from build123d import *

# Parameters (mm, degrees)
F0_W         = 10.668002069
F0_H         = 8.5344007239
F1_DEPTH     = 25.4
F2_W         = 22.2503971308
F2_H         = 8.5344007239
F2_W_2       = 10.668002069
F3_DEPTH     = 10.16
F4_T1_DEPTH  = 80.5687963307
F4_T3_DEPTH  = 34.9503971308
F4_T5_DEPTH  = 34.9503971308
F4_T10_DEPTH = 47.6503971308
F4_T15_DEPTH = 47.6503971308
F4_T20_DEPTH = 47.6503971308
F4_T25_DEPTH = 47.6503971308


# Not quite as in the source:
# - a fillet or chamfer that OpenCascade refuses, or shapes differently, is made with other operations: its cross-section is extruded or revolved along the edge and cut away or added


with BuildPart() as f1:
    # F0 (on Front) → F1 (new body)
    with BuildSketch(Plane.XZ):
        Rectangle(F0_W, F0_H)
    extrude(amount=F1_DEPTH)

    # F2 (on face) → F3 (join)
    with BuildSketch(Plane(origin=(0, 0, 0), x_dir=(-1, 0, 0), z_dir=(0, 1, 0))):
        with Locations((-16.4591995999, 0)):
            Rectangle(F2_W, F2_H)
        Rectangle(F2_W_2, F2_H)
        with Locations((16.4591995999, 0)):
            Rectangle(F2_W, F2_H)
    extrude(amount=F3_DEPTH)

    # F4: fillet of radius 5.08 on 6 edges, made by hand

    # F4_s2 → F4_t1 (cut)
    with BuildSketch(Plane.YZ.offset(-40.2843981653)):
        with BuildLine():
            ThreePointArc((10.16, -0.8127996381), (8.6721024484, 2.7793028104), (5.08, 4.2672003619))
            Line((5.08, 4.2672003619), (10.16, 4.2672003619))
            Line((10.16, 4.2672003619), (10.16, -0.8127996381))
        make_face()
        with BuildLine():
            ThreePointArc((5.08, -4.2672003619), (8.6721024484, -2.7793028104), (10.16, 0.8127996381))
            Line((10.16, 0.8127996381), (10.16, -4.2672003619))
            Line((10.16, -4.2672003619), (5.08, -4.2672003619))
        make_face()
    extrude(amount=F4_T1_DEPTH, mode=Mode.SUBTRACT)

    # F4_s4 → F4_t3 (cut)
    with BuildSketch(Plane.YZ.offset(5.3340010345)):
        with BuildLine():
            ThreePointArc((0, -0.8127996381), (1.4878975516, 2.7793028104), (5.08, 4.2672003619))
            Line((5.08, 4.2672003619), (0, 4.2672003619))
            Line((0, 4.2672003619), (0, -0.8127996381))
        make_face()
        with BuildLine():
            ThreePointArc((5.08, -4.2672003619), (1.4878975516, -2.7793028104), (0, 0.8127996381))
            Line((0, 0.8127996381), (0, -4.2672003619))
            Line((0, -4.2672003619), (5.08, -4.2672003619))
        make_face()
    extrude(amount=F4_T3_DEPTH, mode=Mode.SUBTRACT)

    # F4_s6 → F4_t5 (cut)
    with BuildSketch(Plane.YZ.offset(-40.2843981653)):
        with BuildLine():
            ThreePointArc((5.08, -4.2672003619), (1.4878975516, -2.7793028104), (0, 0.8127996381))
            Line((0, 0.8127996381), (0, -4.2672003619))
            Line((0, -4.2672003619), (5.08, -4.2672003619))
        make_face()
        with BuildLine():
            ThreePointArc((0, -0.8127996381), (1.4878975516, 2.7793028104), (5.08, 4.2672003619))
            Line((5.08, 4.2672003619), (0, 4.2672003619))
            Line((0, 4.2672003619), (0, -0.8127996381))
        make_face()
    extrude(amount=F4_T5_DEPTH, mode=Mode.SUBTRACT)


with BuildPart() as f4_tool8:
    # F4_s9 → F4_t10 (new body)
    with BuildSketch(Plane.YZ.offset(-7.3659989655)):
        with BuildLine():
            ThreePointArc((0, -0.8127996381), (1.4878975516, 2.7793028104), (5.08, 4.2672003619))
            Line((5.08, 4.2672003619), (0, 4.2672003619))
            Line((0, 4.2672003619), (0, -0.8127996381))
        make_face()
    extrude(amount=F4_T10_DEPTH)

    split(bisect_by=Plane.YZ.offset(-5.3340010345), keep=Keep.BOTTOM)


with BuildPart() as f1_1:
    add(f1.part)

    # F4_t7: cut F4_tool8
    add(f4_tool8.part, mode=Mode.SUBTRACT)


with BuildPart() as f4_tool13:
    # F4_s14 → F4_t15 (new body)
    with BuildSketch(Plane.YZ.offset(40.2843981653)):
        with BuildLine():
            ThreePointArc((5.08, -4.2672003619), (1.4878975516, -2.7793028104), (0, 0.8127996381))
            Line((0, 0.8127996381), (0, -4.2672003619))
            Line((0, -4.2672003619), (5.08, -4.2672003619))
        make_face()
    extrude(amount=-F4_T15_DEPTH)

    split(bisect_by=Plane.YZ.offset(-5.3340010345), keep=Keep.BOTTOM)


with BuildPart() as f1_2:
    add(f1_1.part)

    # F4_t12: cut F4_tool13
    add(f4_tool13.part, mode=Mode.SUBTRACT)


with BuildPart() as f4_tool18:
    # F4_s19 → F4_t20 (new body)
    with BuildSketch(Plane.YZ.offset(7.3659989655)):
        with BuildLine():
            ThreePointArc((5.08, -4.2672003619), (1.4878975516, -2.7793028104), (0, 0.8127996381))
            Line((0, 0.8127996381), (0, -4.2672003619))
            Line((0, -4.2672003619), (5.08, -4.2672003619))
        make_face()
    extrude(amount=-F4_T20_DEPTH)

    split(bisect_by=Plane.YZ.offset(5.3340010345), keep=Keep.TOP)


with BuildPart() as f1_3:
    add(f1_2.part)

    # F4_t17: cut F4_tool18
    add(f4_tool18.part, mode=Mode.SUBTRACT)


with BuildPart() as f4_tool23:
    # F4_s24 → F4_t25 (new body)
    with BuildSketch(Plane.YZ.offset(-40.2843981653)):
        with BuildLine():
            ThreePointArc((0, -0.8127996381), (1.4878975516, 2.7793028104), (5.08, 4.2672003619))
            Line((5.08, 4.2672003619), (0, 4.2672003619))
            Line((0, 4.2672003619), (0, -0.8127996381))
        make_face()
    extrude(amount=F4_T25_DEPTH)

    split(bisect_by=Plane.YZ.offset(5.3340010345), keep=Keep.TOP)


with BuildPart() as f1_4:
    add(f1_3.part)

    # F4_t22: cut F4_tool23
    add(f4_tool23.part, mode=Mode.SUBTRACT)


solid = f1_4.part
Part model, mm, in its own coordinate system. Give positions to 0.01 mm unless a question says otherwise; leave off trailing zeros. Order: outer loops, then holes, each group sorted by start corner. A loop starts at its lowest first (then second) coordinate and runs counter-clockwise, first axis right, second up. Notation, with made-up numbers: (46, 56.5) - (104, 56.5) arc R11 cw to (104, 69.5) - close; hole circle Ø8 at (-33, -3). An arc over 180 degrees is marked (long way). Use a Markdown table: item, result.
1) Saw through at C-C on y = -7. List the corners of the cut face in (x, z), plus the area to 3 significant figures.
Checked values:
| item | result |
|---|---|
| outline | (-5.33, -4.27) - (5.33, -4.27) - (5.33, 4.27) - (-5.33, 4.27) - close |
| area | 91.0 mm² |
2) Saw through at A-A on z = 3. List the corners of the cut face in (x, y).
Checked values:
| item | result |
|---|---|
| outline | (-27.58, 1.72) - (-5.33, 1.72) - (-5.33, -25.4) - (5.33, -25.4) - (5.33, 1.72) - (27.58, 1.72) - (27.58, 8.44) - (-27.58, 8.44) - close |
3) Probe L1, parallel to X at y = -9, z = -3.25; L2, parallel to Y at x = -10.5, z = -1; L3, parallel to Y at x = -20.5, z = 0.5. List the from-to ranges inside material, lowest first. Write a range as from..to.
Checked values:
| item | result |
|---|---|
| L1 | -5.33..5.33 |
| L2 | 0.33..9.83 |
| L3 | 0.17..9.99 |
4) Flat gauge pins, fed straight in: P1, Ø2.5, axis at y = -12.5, z = -1.5, coming from the -X side; P2, Ø3, axis at x = 15, z = -1.5, coming from the -Y side; P3, Ø1.5, axis at y = -12, z = -1.5, coming from the +X side. Where does each tip first touch, or does it go through?
Checked values:
| item | result |
|---|---|
| P1 | x = -5.33 |
| P2 | y = 0.07 |
| P3 | x = 5.33 |
5) Saw through at D-D on z = -2. List the corners of the cut face in (x, y).
Checked values:
| item | result |
|---|---|
| outline | (-27.58, 0.85) - (-5.33, 0.85) - (-5.33, -25.4) - (5.33, -25.4) - (5.33, 0.85) - (27.58, 0.85) - (27.58, 9.31) - (-27.58, 9.31) - close |
6) Saw through at B-B on x = 1. List the corners of the cut face in (y, z), plus the area to 3 significant figures.
Checked values:
| item | result |
|---|---|
| outline | (-25.4, -4.27) - (5.08, -4.27) arc R5.08 ccw to (10.09, 0) arc R5.08 ccw to (5.08, 4.27) - (-25.4, 4.27) - close |
| area | 292 mm² |
